from build123d import *

# Parameters (mm, degrees)
F1_DEPTH = 80
F3_DEPTH = 3
F4_R     = 1.65
F5_DEPTH = 3
F6_R     = 11.5
F6_R_2   = 1.65
F6_R_3   = 2.75
F7_DEPTH = 3


# Not quite as in the source:
# - ends of sketch curves that miss each other by under 0.0002 mm in the source are joined


with BuildPart() as f1:
    # F0 (on Front) → F1 (new body)
    with BuildSketch(Plane.XZ):
        with BuildLine():
            ThreePointArc((-35.747114317, -2.25), (-34.1, -0.602885683), (-31.85, 0))
            Line((-31.85, 0), (31.85, 0))
            ThreePointArc((31.85, 0), (34.1, -0.602885683), (35.747114317, -2.25))
            Line((35.747114317, -2.25), (59.047114317, -42.6067838164))
            Line((59.047114317, -42.6067838164), (60.7791651246, -41.6067838164))
            Line((60.7791651246, -41.6067838164), (37.4791651246, -1.25))
            ThreePointArc((37.4791651246, -1.25), (35.1, 1.1291651246), (31.85, 2))
            Line((31.85, 2), (-31.85, 2))
            ThreePointArc((-31.85, 2), (-35.1, 1.1291651246), (-37.4791651246, -1.25))
            Line((-37.4791651246, -1.25), (-60.7791651246, -41.6067838164))
            Line((-60.7791651246, -41.6067838164), (-59.047114317, -42.6067838164))
            Line((-59.047114317, -42.6067838164), (-35.747114317, -2.25))
        make_face()
    extrude(amount=F1_DEPTH)

    # F2 (on face) → F3 (cut)
    with BuildSketch(Plane(origin=(27.5681079661, 0, 15.9164545553), x_dir=(0, 1, 0), z_dir=(0.8660254038, 0, 0.5))):
        with BuildLine():
            Line((-20, -66.422114317), (-20, -28.8756559143))
            ThreePointArc((-20, -28.8756559143), (-40, -8.8756559143), (-60, -28.8756559143))
            Line((-60, -28.8756559143), (-60, -66.422114317))
            Line((-60, -66.422114317), (-20, -66.422114317))
        make_face()
        with BuildLine():
            Line((-72.5, -60.572114317), (-70, -60.572114317))
            ThreePointArc((-70, -60.572114317), (-68.35, -58.922114317), (-70, -57.272114317))
            Line((-70, -57.272114317), (-72.5, -57.272114317))
            ThreePointArc((-72.5, -57.272114317), (-74.15, -58.922114317), (-72.5, -60.572114317))
        make_face()
        with BuildLine():
            Line((-70.0008798832, -23.522114317), (-72.5008798832, -23.522114317))
            ThreePointArc((-72.5008798832, -23.522114317), (-74.1499997654, -25.1729942001), (-72.499120117, -26.8221140824))
            Line((-72.499120117, -26.8221140824), (-69.9991201168, -26.822114317))
            ThreePointArc((-69.9991201168, -26.822114317), (-68.3500002346, -25.171234434), (-70.0008798832, -23.522114317))
        make_face()
        with BuildLine():
            Line((-9.9999995409, -26.822114317), (-7.4999995409, -26.822114317))
            ThreePointArc((-7.4999995409, -26.822114317), (-5.85, -25.1721140875), (-7.5, -23.522114317))
            Line((-7.5, -23.522114317), (-10, -23.522114317))
            ThreePointArc((-10, -23.522114317), (-11.6499997705, -25.1721145466), (-9.9999995409, -26.822114317))
        make_face()
        with BuildLine():
            Line((-10, -60.572114317), (-7.5, -60.572114317))
            ThreePointArc((-7.5, -60.572114317), (-5.85, -58.922114317), (-7.5, -57.272114317))
            Line((-7.5, -57.272114317), (-10, -57.272114317))
            ThreePointArc((-10, -57.272114317), (-11.65, -58.922114317), (-10, -60.572114317))
        make_face()
    extrude(amount=-F3_DEPTH, mode=Mode.SUBTRACT)

    # F4 (on face) → F5 (cut)
    with BuildSketch(Plane(origin=(-27.5681079661, 0, 15.9164545553), x_dir=(0, -1, 0), z_dir=(-0.8660254038, 0, 0.5))):
        with BuildLine():
            Line((20, -56.422114317), (60, -56.422114317))
            ThreePointArc((60, -56.422114317), (40, -36.422114317), (20, -56.422114317))
        make_face()
        with BuildLine():
            Line((60, -66.422114317), (60, -56.422114317))
            ThreePointArc((60, -56.422114317), (59.3185165258, -61.5984952191), (57.3205080757, -66.422114317))
            Line((57.3205080757, -66.422114317), (60, -66.422114317))
        make_face()
        with BuildLine():
            ThreePointArc((57.3205080757, -66.422114317), (59.3185165258, -61.5984952191), (60, -56.422114317))
            Line((60, -56.422114317), (20, -56.422114317))
            ThreePointArc((20, -56.422114317), (20.6814834742, -61.5984952191), (22.6794919243, -66.422114317))
            Line((22.6794919243, -66.422114317), (57.3205080757, -66.422114317))
        make_face()
        with BuildLine():
            ThreePointArc((22.6794919243, -66.422114317), (20.6814834742, -61.5984952191), (20, -56.422114317))
            Line((20, -56.422114317), (20, -66.422114317))
            Line((20, -66.422114317), (22.6794919243, -66.422114317))
        make_face()
        with BuildLine():
            ThreePointArc((22.6794919243, -66.422114317), (40, -76.422114317), (57.3205080757, -66.422114317))
            Line((57.3205080757, -66.422114317), (22.6794919243, -66.422114317))
        make_face()
        with Locations((70, -58.922114317)):
            Circle(F4_R)
        with Locations((69.7541560233, -25.172114317)):
            Circle(F4_R)
        with Locations((10, -58.922114317)):
            Circle(F4_R)
        with Locations((10, -25.172114317)):
            Circle(F4_R)
    extrude(amount=-F5_DEPTH, mode=Mode.SUBTRACT)

    # F6 (on face) → F7 (cut)
    with BuildSketch(Plane.XY.offset(2)):
        with Locations((0, -40)):
            Circle(F6_R)
        with Locations((-15, -5)):
            Circle(F6_R_2)
        with Locations((0, -5)):
            Circle(F6_R_2)
        with Locations((15, -5)):
            Circle(F6_R_2)
        with Locations((-10, -13.93)):
            Circle(F6_R_3)
        with Locations((0, -13.93)):
            Circle(F6_R_3)
        with Locations((10, -13.93)):
            Circle(F6_R_3)
        with Locations((-10, -66.07)):
            Circle(F6_R_3)
        with Locations((0, -66.07)):
            Circle(F6_R_3)
        with Locations((10, -66.07)):
            Circle(F6_R_3)
        with Locations((0, -75)):
            Circle(F6_R_2)
        with Locations((-15, -75)):
            Circle(F6_R_2)
        with Locations((15, -75)):
            Circle(F6_R_2)
        with BuildLine():
            Line((-18.4225551057, -63.817408691), (-21.9925551057, -61.317408691))
            ThreePointArc((-21.9925551057, -61.317408691), (-25.822591309, -61.9925551057), (-25.1474448943, -65.822591309))
            Line((-25.1474448943, -65.822591309), (-21.5774448943, -68.322591309))
            ThreePointArc((-21.5774448943, -68.322591309), (-17.747408691, -67.6474448943), (-18.4225551057, -63.817408691))
        make_face()
        with BuildLine():
            Line((-21.5774448943, -11.677408691), (-25.1474448943, -14.177408691))
            ThreePointArc((-25.1474448943, -14.177408691), (-25.822591309, -18.0074448943), (-21.9925551057, -18.682591309))
            Line((-21.9925551057, -18.682591309), (-18.4225551057, -16.182591309))
            ThreePointArc((-18.4225551057, -16.182591309), (-17.747408691, -12.3525551057), (-21.5774448943, -11.677408691))
        make_face()
        with BuildLine():
            Line((25.1474448943, -14.177408691), (21.5774448943, -11.677408691))
            ThreePointArc((21.5774448943, -11.677408691), (17.747408691, -12.3525551057), (18.4225551057, -16.182591309))
            Line((18.4225551057, -16.182591309), (21.9925551057, -18.682591309))
            ThreePointArc((21.9925551057, -18.682591309), (25.822591309, -18.0074448943), (25.1474448943, -14.177408691))
        make_face()
        with BuildLine():
            Line((21.9925551057, -61.317408691), (18.4225551057, -63.817408691))
            ThreePointArc((18.4225551057, -63.817408691), (17.747408691, -67.6474448943), (21.5774448943, -68.322591309))
            Line((21.5774448943, -68.322591309), (25.1474448943, -65.822591309))
            ThreePointArc((25.1474448943, -65.822591309), (25.822591309, -61.9925551057), (21.9925551057, -61.317408691))
        make_face()
        with BuildLine():
            Line((-11.833273811, -25.833273811), (-14.333273811, -23.333273811))
            ThreePointArc((-14.333273811, -23.333273811), (-16.666726189, -23.333273811), (-16.666726189, -25.666726189))
            Line((-16.666726189, -25.666726189), (-14.166726189, -28.166726189))
            ThreePointArc((-14.166726189, -28.166726189), (-11.833273811, -28.166726189), (-11.833273811, -25.833273811))
        make_face()
        with BuildLine():
            Line((-14.333273811, -56.666726189), (-11.833273811, -54.166726189))
            ThreePointArc((-11.833273811, -54.166726189), (-11.833273811, -51.833273811), (-14.166726189, -51.833273811))
            Line((-14.166726189, -51.833273811), (-16.666726189, -54.333273811))
            ThreePointArc((-16.666726189, -54.333273811), (-16.666726189, -56.666726189), (-14.333273811, -56.666726189))
        make_face()
        with BuildLine():
            Line((16.666726189, -54.333273811), (14.166726189, -51.833273811))
            ThreePointArc((14.166726189, -51.833273811), (11.833273811, -51.833273811), (11.833273811, -54.166726189))
            Line((11.833273811, -54.166726189), (14.333273811, -56.666726189))
            ThreePointArc((14.333273811, -56.666726189), (16.666726189, -56.666726189), (16.666726189, -54.333273811))
        make_face()
        with BuildLine():
            Line((14.333273811, -23.333273811), (11.833273811, -25.833273811))
            ThreePointArc((11.833273811, -25.833273811), (11.833273811, -28.166726189), (14.166726189, -28.166726189))
            Line((14.166726189, -28.166726189), (16.666726189, -25.666726189))
            ThreePointArc((16.666726189, -25.666726189), (16.666726189, -23.333273811), (14.333273811, -23.333273811))
        make_face()
    extrude(amount=-F7_DEPTH, mode=Mode.SUBTRACT)


solid = f1.part
Check sheet for the modelled part. Datum: model origin and axes. Units: mm. A direction names the side the tool comes from. Give positions to 0.01 mm unless a question says otherwise; leave off trailing zeros. Order: outer loops, then holes, each group sorted by start corner. A loop starts at its lowest first (then second) coordinate and runs counter-clockwise, first axis right, second up. Notation, with made-up numbers: M 67.25,-16.5 L 79.25,-16.5 A15 ccw 79.25,8.5 Z; hole C 4.25,56.25 d8. An arc over 180 degrees is marked long. Answer as CSV lines item,"result". Start each with the question number.
Item 1: Mould release check, pull along Y, two halves, no side actions. Record for faces 1 (the face through (8, -31, 2)), 2 (the face through (25.787, -18.057, 1.014)): +Y half, -Y half, draft (parallel to the pull), parting line (faces both ways), or undercut.
Item 2: Cross-section at B-B on y = -37. Enter the section's corners in (x, z), plus the area to 3 significant figures.
Item 3: Cross-section at C-C on x = -5. Enter the section's corners in (y, z), plus the area to 3 significant figures.
Item 4: Thickness scan on line 1 (Y direction, x = 0, z = 1); line 2 (X direction, y = -16, z = 0.5); line 3 (X direction, y = -75, z = 0.65). Record the ranges inside material, lowest first. Write a range as [from, to].
Item 5: Cross-section at A-A on x = 10. Enter the section's corners in (y, z).
Item 6: Tool access check on faces 3 (the face through (20.23, -62.55, 1.01)), 4 (the face through (39.28, -11.65, -6.34)), 5 (the face through (-34.13, -39.44, -0.62)). Record the directions out of +Z, -Z, +X, -X, +Y, -Y that give a thin tool (end or side, any length) a straight path to the whole face; none if there is none.
Item 7: Cross-section at D-D on x = -23.57. Enter the section's corners in (y, z), plus the area to 3 significant figures.
Item 8: Gauge pin test, flat ends, axial feed: P1, Ø3, axis at x = 11, y = -42.5, coming from the -Z side; P2, Ø8, axis at y = -22, z = -36.5, coming from the +X side; P3, Ø1, axis at y = -8.5, z = -22.5, coming from the -X side; P4, Ø3.5, axis at x = 0, y = -66.07, coming from the -Z side. Record the tip position at first contact, or that the pin passes through.
Established:
1,face 1,"draft"
1,face 2,"undercut"
2,outline,"M -45.89,-15.82 L -44.16,-16.82 L -35.75,-2.25 A4.5 cw -31.85,0 L -11.1,0 L -11.1,2 L -31.85,2 A6.5 ccw -37.48,-1.25 Z; M 11.1,0 L 31.85,0 A4.5 cw 33.47,-0.3 L 32.14,1.99 A6.5 ccw 31.85,2 L 11.1,2 Z"
2,area,"130 mm^2"
3,outline,"M -80,0 L -50.36,0 L -50.36,2 L -80,2 Z; M -29.64,0 L 0,0 L 0,2 L -29.64,2 Z"
3,area,"119 mm^2"
4,line 1,"y = [-80, -76.65], [-73.35, -68.82], [-63.32, -51.5], [-28.5, -16.68], [-11.18, -6.65], [-3.35, 0]"
4,line 2,"x = [-36, -26.29], [-18.19, -11.81], [-8.19, -1.81], [1.81, 8.19], [11.81, 18.19], [26.29, 36]"
4,line 3,"x = [-35.82, -16.65], [-13.35, -1.65], [1.65, 13.35], [16.65, 35.82]"
5,outline,"M -80,0 L -68.82,0 L -68.82,2 L -80,2 Z; M -63.32,0 L -45.68,0 L -45.68,2 L -63.32,2 Z; M -34.32,0 L -16.68,0 L -16.68,2 L -34.32,2 Z; M -11.18,0 L 0,0 L 0,2 L -11.18,2 Z"
6,face 3,"+Z, -Z"
6,face 4,"none"
6,face 5,"-Z, +Y, -Y"
7,outline,"M -80,0 L -66.93,0 L -66.93,2 L -80,2 Z; M -60.82,0 L -19.18,0 L -19.18,2 L -60.82,2 Z; M -13.07,0 L 0,0 L 0,2 L -13.07,2 Z"
7,area,"136 mm^2"
8,P1,"stops at z = 0"
8,P2,"stops at x = 59.83"
8,P3,"stops at x = -50.04"
8,P4,"passes through"
